Could you check a few things on this model? Use its own coordinates, in mm. A direction names the side the tool comes from. Round coordinates to 2 decimals unless told otherwise and drop trailing zeros. Loops run counter-clockwise (first coordinate to the right, second up) from the corner with the lowest first, then second, coordinate; pieces in that order, holes last. Notation, with made-up numbers: (59, -27.75) -> (117, -27.75) arc R21 cw to (117, -17.75) -> close; hole circle Ø1 at (73, 11). An arc over 180 degrees is marked (long way). One line per item, written item: value.
```python
from build123d import *

# Parameters (mm, degrees)
F0_W     = 296.7444360256
F0_H     = 164.8739129305
F0_R     = 20.7617734551
F0_R_2   = 23.6179830604
F1_DEPTH = 104.394
F3_DEPTH = 25.4
F5_DEPTH = 25.4
F6_DEPTH = 237.998


with BuildPart() as f1:
    # F0 (on Top) → F1 (new body)
    with BuildSketch(Plane.XY):
        Rectangle(F0_W, F0_H)
        with Locations((-108.6655110121, 0)):
            Circle(F0_R, mode=Mode.SUBTRACT)
        with Locations((109.9524945021, 0)):
            Circle(F0_R_2, mode=Mode.SUBTRACT)
    extrude(amount=F1_DEPTH)

    # F2 (on face) → F3 (join)
    with BuildSketch(Plane.XZ.offset(82.4369564652)):
        with BuildLine():
            ThreePointArc((-69.8260508727, 104.394), (0, 34.5679491273), (69.8260508727, 104.394))
            Line((69.8260508727, 104.394), (54.0751636947, 104.394))
            ThreePointArc((54.0751636947, 104.394), (0, 50.3188363053), (-54.0751636947, 104.394))
            Line((-54.0751636947, 104.394), (-69.8260508727, 104.394))
        make_face()
    extrude(amount=F3_DEPTH)

    # F4 (on face) → F5 (join)
    with BuildSketch(Plane(origin=(0, 82.4369564652, 0), x_dir=(-1, 0, 0), z_dir=(0, 1, 0))):
        with BuildLine():
            Line((64.3801944151, 104.394), (53.3518843102, 104.394))
            ThreePointArc((53.3518843102, 104.394), (0, 51.0421156898), (-53.3518843102, 104.394))
            Line((-53.3518843102, 104.394), (-64.3801944151, 104.394))
            ThreePointArc((-64.3801944151, 104.394), (0, 40.0138055849), (64.3801944151, 104.394))
        make_face()
    extrude(amount=F5_DEPTH)

    # F6 (cut): a face of the model
    f6_faces = [f1.faces().sort_by_distance(p)[0] for p in [
        (0, -82.4369564652, 81.443787732),
    ]]
    extrude(f6_faces, amount=-F6_DEPTH, mode=Mode.SUBTRACT)


solid = f1.part
```
(1) Imagine slicing it at B-B on x = 94. Write out the boundary of the cut face in (y, z), then the cut area to 3 significant figures.
Results below:
outline: (-82.44, 0) -> (-17.42, 0) -> (-17.42, 104.39) -> (-82.44, 104.39) -> close; (17.42, 0) -> (82.44, 0) -> (82.44, 104.39) -> (17.42, 104.39) -> close
area: 13,600 mm²
(2) Imagine slicing it at A-A on y = 0. Write out the boundary of the cut face in (x, z), then the cut area to 3 significant figures.
Results below:
outline: (-148.37, 0) -> (-129.43, 0) -> (-129.43, 104.39) -> (-148.37, 104.39) -> close; (-87.9, 0) -> (86.33, 0) -> (86.33, 104.39) -> (54.08, 104.39) arc R54.08 cw to (-54.08, 104.39) -> (-87.9, 104.39) -> close; (133.57, 0) -> (148.37, 0) -> (148.37, 104.39) -> (133.57, 104.39) -> close
area: 17,100 mm²
(3) On a 3-axis mill with a long thin cutter (end or side, diameter ignored), from which of +Z, -Z, +X, -X, +Y, -Y can I reach the whole of each face in a straight line? I mean faces 1 (the face through (-1.535, -94.959, 34.585)), 2 (the face through (1.42, 94.96, 40.03)), 3 (the face through (1.19, -1.51, 50.33)). Say none if no direction works.
Results below:
face 1: -Z, -Y
face 2: -Z, +Y
face 3: +Z, +Y, -Y
(4) For pin 1 Ø6 at (x, z) = (74, 56.5) entering from -Y; pin 2 Ø8 at (x, z) = (-88.5, 93.5) entering from +Y, each with a flat end and sliding along its axis, tell me the tip position at first contact or that it passes through.
Results below:
pin 1: stops at y = -82.44
pin 2: stops at y = 82.44
(5) Please list where these lines run through material, in increasing order: L1, parallel to X at y = 54, z = 87; L2, parallel to Y at x = -131, z = 46.5; L3, parallel to X at y = -9, z = 10.
Results below:
L1: x = -148.37 to -51.2, 51.2 to 148.37
L2: y = -82.44 to 82.44
L3: x = -148.37 to -127.38, -89.96 to 88.12, 131.79 to 148.37
(6) We'd pull the mould along Y, two halves only. Please class faces 4 (the face through (-129.407, 0.913, 51.466)), 5 (the face through (-2.08, 82.437, 39.87)), 6 (the face through (148.372, -1, 51)): +Y half, -Y half, draft (parallel to the pull), parting line (faces both ways), or undercut.
Results below:
face 4: undercut
face 5: +Y half
face 6: draft
(7) Imagine slicing it at C-C on z = 31. Write out the boundary of the cut face in (x, y), then the cut area to 3 significant figures.
Results below:
outline: (-148.37, -82.44) -> (148.37, -82.44) -> (148.37, 82.44) -> (-148.37, 82.44) -> close; hole circle Ø41.52 at (-108.67, 0); hole circle Ø47.24 at (109.95, 0)
area: 45,800 mm²
(8) Imagine slicing it at D-D on x = 0. Write out the boundary of the cut face in (y, z).
Results below:
outline: (-107.84, 34.57) -> (-82.44, 34.57) -> (-82.44, 0) -> (82.44, 0) -> (82.44, 40.01) -> (107.84, 40.01) -> (107.84, 50.32) -> (-107.84, 50.32) -> close
